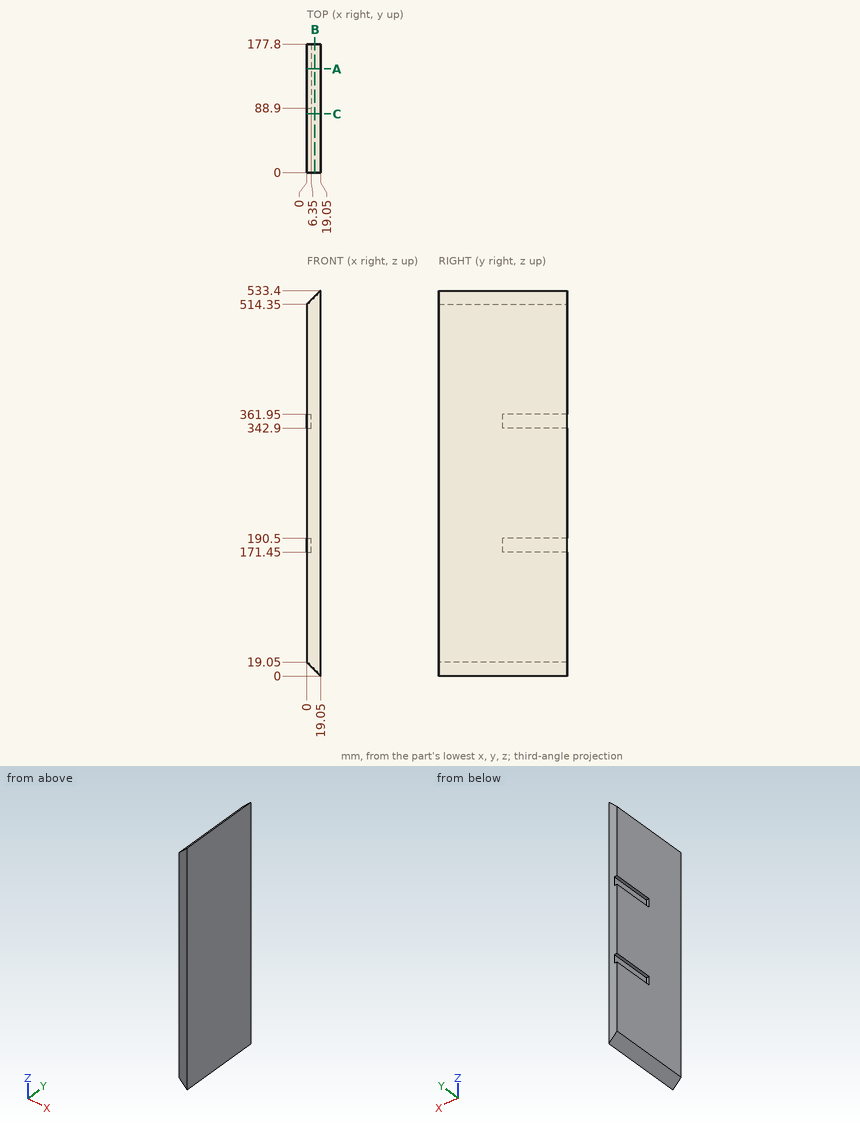
Verification items for this drawing (mm, ordinates from the low corner). Coordinates: 2 decimals unless noted, no trailing zeros. Loops run counter-clockwise (first coordinate to the right, second up) from the corner with the lowest first, then second, coordinate; pieces in that order, holes last. Notation, with made-up numbers: (69.5, 57) -> (86.5, 57) arc R22 cw to (86.5, 74) -> close; hole circle Ø7 at (82, 88.5). An arc over 180 degrees is marked (long way). Put each result on its own line as item: value.
1. Section check C-C, the plane y = 81. Record the boundary of the cut face in (x, z).
Result set:
outline: (0, 19.05) -> (19.05, 0) -> (19.05, 533.4) -> (0, 514.35) -> close
2. Section check A-A, the plane y = 143.5. Record the boundary of the cut face in (x, z).
Result set:
outline: (0, 19.05) -> (19.05, 0) -> (19.05, 533.4) -> (0, 514.35) -> (0, 361.95) -> (6.35, 361.95) -> (6.35, 342.9) -> (0, 342.9) -> (0, 190.5) -> (6.35, 190.5) -> (6.35, 171.45) -> (0, 171.45) -> close
3. Section check B-B, the plane x = 11. Record the boundary of the cut face in (y, z).
Result set:
outline: (0, 8.05) -> (177.8, 8.05) -> (177.8, 525.35) -> (0, 525.35) -> close
4. Thickness scan on line 1 (Z direction, x = 3, y = 120); line 2 (Z direction, x = 3.25, y = 124.5); line 3 (Z direction, x = 5.25, y = 58.5). Record the ranges inside material, lowest first.
Result set:
line 1: z = 16.05 to 171.45, 190.5 to 342.9, 361.95 to 517.35
line 2: z = 15.8 to 171.45, 190.5 to 342.9, 361.95 to 517.6
line 3: z = 13.8 to 519.6
5. Gauge pin test, flat ends, axial feed: P1, Ø7, axis at x = 3, y = 128.5, coming from the -Z side; P2, Ø8, axis at x = 7.5, y = 141, coming from the -Z side; P3, Ø15, axis at y = 139, z = 353.5, coming from the -X side. Record the tip position at first contact, or that the pin passes through.
Result set:
P1: stops at z = 12.55
P2: stops at z = 7.55
P3: stops at x = 6.35
